Source: CAD feature listing. Evaluate the final solid. Frame: model axes, mm. A direction names the side the tool comes from. Give positions to 0.01 mm unless a question says otherwise; leave off trailing zeros. Write each loop counter-clockwise with the first axis right and the second up, starting at its lowest first coordinate (ties: lowest second). Pieces come first, ordered by that corner, then holes. Notation, with made-up numbers: M 13.5,-39.5 L 41.5,-39.5 A15 cw 41.5,-12.5 Z; hole C 25,-17.75 d6. An arc over 180 degrees is marked long. Answer as a JSON object with one key per item and string values. Group by question number.
Autodesk Inventor part; units mm, degrees
ref_plane "YZ Plane" through (0, 0, 0) normal (1, 0, 0) x (0, 1, 0)
ref_plane "XZ Plane" through (0, 0, 0) normal (0, 1, 0) x (-1, 0, 0)
ref_plane "XY Plane" through (0, 0, 0) normal (0, 0, 1) x (1, 0, 0)
sketch "Boceto1" plane through (0, 0, 0) normal (0, 1, 0) x (-1, 0, 0)
  circle A0 centre (0, 0) radius 6.8
  circle A1 centre (0, 0) radius 6.1
  dimension "d0" = 13.6
  dimension "d1" = 12.2
extrude "Extrusión1" add sketch "Boceto1" against normal blind 1.5
sketch "Boceto2" plane through (0, -1.5, 0) normal (0, -1, 0) x (1, 0, 0)
  circle A0 centre (0, 0) radius 6.7588
  circle A1 centre (0, 0) radius 8.2
  dimension "d4" = 16.4
extrude "Extrusión2" add sketch "Boceto2" along normal blind 1.4
properties part number "Elemento_externo" material "Plástico ABS"
(1) Ray query, L1, parallel to X at y = -1.7, z = 0.25; L2, parallel to Z at x = 0, y = -2.15; L3, parallel to Z at x = 0, y = -0.85. Return the intervals inside material, ascending. Write a range as [from, to].
(2) Section D-D, the plane y = -2.55. Return loops of the section in (x, z), plus the area to 3 significant figures.
(3) Section C-C, the plane y = -0.65. Return loops of the section in (x, z), plus the area to 3 significant figures.
(4) Section B-B, the plane z = 0. Return loops of the section in (x, y), plus the area to 3 significant figures.
(5) Contact query for flat-ended pins moving along their axis: pin 1 Ø4 at (x, z) = (-1.5, 2.5) entering from -Y; pin 2 Ø1 at (x, y) = (3.5, -1.5) entering from +Z; pin 3 Ø1.5 at (x, y) = (-1, -1.5) entering from -Z. Output: stop coordinate, or through.
(6) Section A-A, the plane x = 0. Return loops of the section in (y, z), plus the area to 3 significant figures.
(7) Access query for faces 4 (the cylindrical face through (6.447, -2.19, -2.03)), 5 (the flat face through (1, -1.5, 7)), 6 (the cylindrical face through (6.094, -0.74, 0.268)). Directions: +Z, -Z, +X, -X, +Y, -Y. A direction counts if a zero-diameter tool reaches every point of the face in a straight line with its end or side. Return the directions, or none.
(8) Pull-direction query (Z, two-part tool) for faces 1 (the cylindrical face through (1.47, -0.74, -6.64)), 2 (the flat face through (1, -2.9, 7)), 3 (the flat face through (4, -1.5, 5)); classes: pulls with the +Z half, pulls with the -Z half, needs draft (parallel to the pull), parting line crosses it, or undercut.
Reported:
{
 "1": {"L1": "x = [-8.2, -6.75], [6.75, 8.2]", "L2": "z = [-8.2, -6.76], [6.76, 8.2]", "L3": "z = [-6.8, -6.1], [6.1, 6.8]"},
 "2": {"outline": "C 0,0 d16.4; hole C 0,0 d13.52", "area": "67.7 mm2"},
 "3": {"outline": "C 0,0 d13.6; hole C 0,0 d12.2", "area": "28.4 mm2"},
 "4": {"outline": "M -8.2,-2.9 L -6.76,-2.9 L -6.76,-1.5 L -6.1,-1.5 L -6.1,0 L -6.8,0 L -6.8,-1.5 L -8.2,-1.5 Z; M 6.1,-1.5 L 6.76,-1.5 L 6.76,-2.9 L 8.2,-2.9 L 8.2,-1.5 L 6.8,-1.5 L 6.8,0 L 6.1,0 Z", "area": "6.14 mm2"},
 "5": {"pin 1": "passes through", "pin 2": "stops at z = 7.63", "pin 3": "stops at z = -8.2"},
 "6": {"outline": "M -2.9,-8.2 L -1.5,-8.2 L -1.5,-6.8 L 0,-6.8 L 0,-6.1 L -1.5,-6.1 L -1.5,-6.76 L -2.9,-6.76 Z; M -2.9,6.76 L -1.5,6.76 L -1.5,6.1 L 0,6.1 L 0,6.8 L -1.5,6.8 L -1.5,8.2 L -2.9,8.2 Z", "area": "6.14 mm2"},
 "7": {"face 4": "-Y", "face 5": "+Y", "face 6": "+Y, -Y"},
 "8": {"face 1": "parting line crosses it", "face 2": "needs draft", "face 3": "undercut"}
}
